For this review, take the finished solid that the model builds, in its own axes (mm). Face numbers are marked on the shaded views. A direction names the side the tool comes from. Round coordinates to 2 decimals unless told otherwise and drop trailing zeros. Loops run counter-clockwise (first coordinate to the right, second up) from the corner with the lowest first, then second, coordinate; pieces in that order, holes last. Notation, with made-up numbers: (74, 44) -> (85, 44) arc R11 cw to (85, 55) -> close; hole circle Ø3 at (-28, 89). An arc over 180 degrees is marked (long way). One line per question, with ' | ' between items. Start each with the question number.
1. Wall thickness on line 1 along X through (y, z) = (40, -1); line 2 along Z through (x, y) = (-18.5, 37); line 3 along Y through (x, z) = (5.5, -22): over which ranges is each line inside the solid? List them lowest first.
2. Consider section D-D (y = 45.75). Write out the cut boundary in (x, z).
3. Consider section B-B (y = 30.25). Write out the cut boundary in (x, z).
4. Consider section A-A (z = -40). Write out the cut boundary in (x, y), and give its area (3 significant figures).
5. For pin 1 Ø23 at (x, y) = (3.5, 31.5) entering from -Z, flat-tipped, find the tip position at first contact; note if it passes through.
6. Draft analysis for pull direction X (two halves, no side actions). For the marked faces 3, 4 and 5, state which applies: pulls with the +X half, pulls with the -X half, needs draft (parallel to the pull), parting line crosses it, or undercut.
7. Consider section C-C (x = 0). Write out the cut boundary in (y, z), and give its area (3 significant figures).
8. For the marked faces 1 and 2, list the 3-axis set-ups (+Z, -Z, +X, -X, +Y, -Y) from which the entire face can be reached by the end or side of a thin tool; tool diameter is ignored.
```python
from build123d import *

# Parameters (mm, degrees)
EXTRUDE_THIN1_DEPTH = 25
SKETCH2_R           = 11.05
SKETCH2_R_2         = 1.75
CUT_EXTRUDE1_DEPTH  = 79.02002948
CHAMFER1_SIZE       = 4
CUT_EXTRUDE3_DEPTH  = 79.02002948
FILLET1_R           = 2
RIB1_REACH          = 91.231
SKETCH6_WALL_W      = 204.315201322
SKETCH6_WALL_H      = 3


with BuildPart() as part:
    # Sketch1 → Extrude-Thin1 (new, symmetric)
    with BuildSketch(Plane(origin=(0, 0, 0), x_dir=(0, 0, -1), z_dir=(1, 0, 0))):
        Polygon((0, 51.25), (0, 0), (53.25, 0), (53.25, 3), (3, 3), (3, 51.25), align=None)
    extrude(amount=EXTRUDE_THIN1_DEPTH, both=True)

    # Sketch2 → Cut-Extrude1 (cut, through all)
    with BuildSketch(Plane.XY):
        with Locations((0, 30.25)):
            Circle(SKETCH2_R)
        with Locations((-9.898989847, 40.15)):
            Circle(SKETCH2_R_2)
        with Locations((-15.5, 45.75)):
            Circle(SKETCH2_R_2)
        with Locations(Location((9.898989847, 40.15, 0), (0, 0, 90))):
            Circle(SKETCH2_R_2)
        with Locations(Location((15.5, 45.75, 0), (0, 0, 90))):
            Circle(SKETCH2_R_2)
        with Locations((15.5, 14.75)):
            Circle(SKETCH2_R_2)
        with Locations((9.898989847, 20.35)):
            Circle(SKETCH2_R_2)
        with Locations(Location((-9.898989847, 20.35, 0), (0, 0, 90))):
            Circle(SKETCH2_R_2)
        with Locations(Location((-15.5, 14.75, 0), (0, 0, 90))):
            Circle(SKETCH2_R_2)
    extrude(amount=-CUT_EXTRUDE1_DEPTH, mode=Mode.SUBTRACT)

    # Chamfer1
    chamfer1_edges = [part.edges().sort_by_distance(p)[0] for p in [
        (25, 51.25, -1.5),
        (-25, 51.25, -1.5),
        (-25, 1.5, -53.25),
        (25, 1.5, -53.25),
    ]]
    chamfer(chamfer1_edges, length=CHAMFER1_SIZE)

    # Sketch4 → Cut-Extrude3 (cut, through all)
    with BuildSketch(Plane(origin=(0, 0, 0), x_dir=(1, 0, 0), z_dir=(0, 1, 0))):
        with BuildLine():
            Line((-12.9, 41), (-12.9, 11))
            ThreePointArc((-12.9, 11), (-15, 8.9), (-17.1, 11))
            Line((-17.1, 11), (-17.1, 41))
            ThreePointArc((-17.1, 41), (-15, 43.1), (-12.9, 41))
        make_face()
        with BuildLine():
            Line((12.9, 41), (12.9, 11))
            ThreePointArc((12.9, 11), (15, 8.9), (17.1, 11))
            Line((17.1, 11), (17.1, 41))
            ThreePointArc((17.1, 41), (15, 43.1), (12.9, 41))
        make_face()
    extrude(amount=CUT_EXTRUDE3_DEPTH, mode=Mode.SUBTRACT)

    # Fillet1
    fillet1_edges = [part.edges().sort_by_distance(p)[0] for p in [
        (0, 3, -3),
    ]]
    fillet(fillet1_edges, radius=FILLET1_R)

    # Sketch6 wall → Rib1 (add, up to next)
    with BuildSketch(Plane(origin=(25, 13, -9.5), x_dir=(0, -0.838443616301, -0.544988350595), z_dir=(0, 0.544988350595, -0.838443616301)), mode=Mode.PRIVATE) as rib1_sk1:
        with Locations((0, 1.5)):
            Rectangle(SKETCH6_WALL_W, SKETCH6_WALL_H)
    rib1_tool1 = extrude(rib1_sk1.sketch, amount=-RIB1_REACH, mode=Mode.PRIVATE) - part.part
    rib1 = rib1_tool1.solids().sort_by_distance((25, 13, -9.5))[0]
    add(rib1)

    # Mirror1: Rib1 across plane
    add(rib1.mirror(Plane(origin=(0, 0, 0), x_dir=(0, 0, 1), z_dir=(1, 0, 0))))


solid = part.part
```
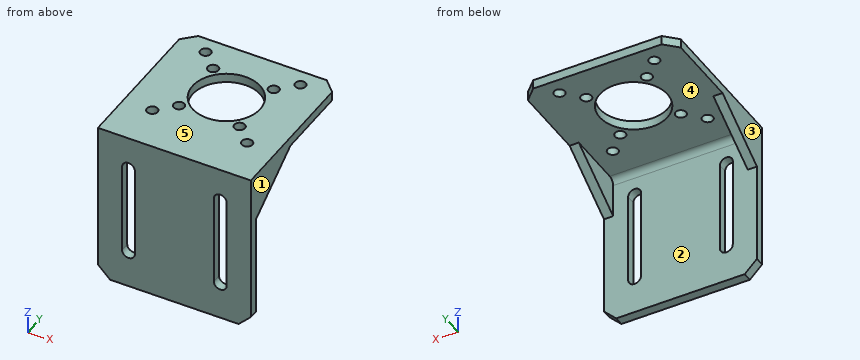
Answer block:
1) line 1: x = -25 to -11.64, -8.16 to -5.2, 5.2 to 8.16, 11.64 to 25 | line 2: z = -3 to 0 | line 3: y = 0 to 3
2) outline: (-25, -3) -> (-17.25, -3) -> (-17.25, 0) -> (-25, 0) -> close; (-13.75, -3) -> (13.75, -3) -> (13.75, 0) -> (-13.75, 0) -> close; (17.25, -3) -> (25, -3) -> (25, 0) -> (17.25, 0) -> close
3) outline: (-25, -3) -> (-11.05, -3) -> (-11.05, 0) -> (-25, 0) -> close; (11.05, -3) -> (25, -3) -> (25, 0) -> (11.05, 0) -> close
4) outline: (-25, 0) -> (-17.1, 0) -> (-17.1, 3) -> (-25, 3) -> close; (-12.9, 0) -> (12.9, 0) -> (12.9, 3) -> (-12.9, 3) -> close; (17.1, 0) -> (25, 0) -> (25, 3) -> (17.1, 3) -> close | area: 125 mm2
5) pin 1: stops at z = -3
6) face 3: pulls with the -X half | face 4: undercut | face 5: needs draft
7) outline: (0, -53.25) -> (3, -53.25) -> (3, -5) arc R2 cw to (5, -3) -> (19.2, -3) -> (19.2, 0) -> (0, 0) -> close; (41.3, -3) -> (51.25, -3) -> (51.25, 0) -> (41.3, 0) -> close | area: 239 mm2
8) face 1: +Z, -Z, +X, +Y, -Y | face 2: -Z, +Y
